```python
from build123d import *

# Parameters (mm, degrees)
BOSS_EXTRUDE1_DEPTH = 660.4
SKETCH2_RX          = 7.33298
SKETCH2_RY          = 7.27642549
CUT_EXTRUDE1_DEPTH  = 33.02
SKETCH3_R           = 32.004
BOSS_EXTRUDE2_DEPTH = 114.6048


with BuildPart() as part:
    # Sketch1 → Boss-Extrude1 (new body)
    with BuildSketch(Plane.XY):
        Polygon((5.802204234, 13.469402687), (-8.763742784, 11.759557608), (-14.565947018, -1.709845079), (-5.802204234, -13.469402687), (8.763742784, -11.759557608), (14.565947018, 1.709845079), align=None)
    extrude(amount=BOSS_EXTRUDE1_DEPTH)

    # Sketch2 → Cut-Extrude1 (cut)
    with BuildSketch(Plane(origin=(-1.480769275, 12.614480148, 0), x_dir=(0.9931806044692795, 0.11658596358926146, 0), z_dir=(-0.11658596358926147, 0.9931806044692796, 0))):
        with Locations(Location((0, -627.66702), (0, 0, 180))):
            Ellipse(SKETCH2_RX, SKETCH2_RY)
    extrude(amount=-CUT_EXTRUDE1_DEPTH, mode=Mode.SUBTRACT)

    # Sketch3 → Boss-Extrude2 (add)
    with BuildSketch(Plane.XY):
        Circle(SKETCH3_R)
    extrude(amount=BOSS_EXTRUDE2_DEPTH)


solid = part.part
```
The listing builds one solid part. Answer for the finished solid, in the listing's coordinates (mm). A direction names the side the tool comes from. Coordinates: 2 decimals unless noted, no trailing zeros. Write each loop counter-clockwise with the first axis right and the second up, starting at its lowest first coordinate (ties: lowest second). Pieces come first, ordered by that corner, then holes. Notation, with made-up numbers: (28, 61) -> (40, 61) arc R21 cw to (40, 76) -> close; hole circle Ø11 at (61.5, -25). An arc over 180 degrees is marked (long way). Write each question's results on one line, items separated by ' | '. Start each with the question number.
1) A tool of negligible diameter and unlimited length cuts with its end or side. For faces 1 (the flat face through (1.379, -12.626, 647.441)), 2 (the flat face through (-11.624, 5.119, 383.682)), 3 (the flat face through (-10.245, -7.507, 383.682)), 4 (the flat face through (0, -14, 114.605)), 5 (the flat face through (10.245, 7.507, 383.682)), from which of +Z, -Z, +X, -X, +Y, -Y can it reach the whole face along a straight path? Write none if from no direction.
2) A cutting plane is placed at A-A (z = 155). Determine the outline of the cut face in (x, y).
3) Straight lines are drawn through the part: probe 1 along Z at (x, y) = (-21.5, 13.5); probe 2 along Z at (x, y) = (-6, -7); probe 3 along Z at (x, y) = (5, -1.5). For each, find the intervals that lie inside material, in ascending order.
4) Flat-ended cylindrical pins translate along their axes: pin 1 Ø1 at (x, z) = (2, 92) entering from -Y; pin 2 Ø1.5 at (x, z) = (-13, 591) entering from -Y; pin 3 Ø2 at (y, z) = (12.5, 343) entering from +X. Find the tip coordinate at first contact, or state that the pin passes through.
5) A cutting plane is placed at B-B (y = 26). Determine the outline of the cut face in (x, z), then the cut area to 3 significant figures.
6) A cutting plane is placed at C-C (y = -24.5). Determine the outline of the cut face in (x, z), then the cut area to 3 significant figures.
Values follow:
1) face 1: +Z, +X, -Y | face 2: +Z, -X, +Y | face 3: +Z, -X, -Y | face 4: +Z | face 5: +Z, +X, +Y
2) outline: (-14.57, -1.71) -> (-5.8, -13.47) -> (8.76, -11.76) -> (14.57, 1.71) -> (5.8, 13.47) -> (-8.76, 11.76) -> close
3) probe 1: 0 to 114.6 | probe 2: 0 to 624.88, 630.45 to 660.4 | probe 3: 0 to 622.16, 633.18 to 660.4
4) pin 1: y = -31.97 | pin 2: y = -4.82 | pin 3: x = 7.27
5) outline: (-18.66, 0) -> (18.66, 0) -> (18.66, 114.6) -> (-18.66, 114.6) -> close | area: 4,280 mm²
6) outline: (-20.59, 0) -> (20.59, 0) -> (20.59, 114.6) -> (-20.59, 114.6) -> close | area: 4,720 mm²
